Print and shaded views of the part. All mm, measured from the part's lowest x, y and z. A direction names the side the tool comes from. Round coordinates to 2 decimals unless told otherwise and drop trailing zeros. Order: outer loops, then holes, each group sorted by start corner. A loop starts at its lowest first (then second) coordinate and runs counter-clockwise, first axis right, second up. Notation, with made-up numbers: (77, 32) -> (123, 32) arc R26 cw to (123, 69) -> close; hole circle Ø1 at (10.5, 68.25). An arc over 180 degrees is marked (long way). Answer as CSV lines item,"result".
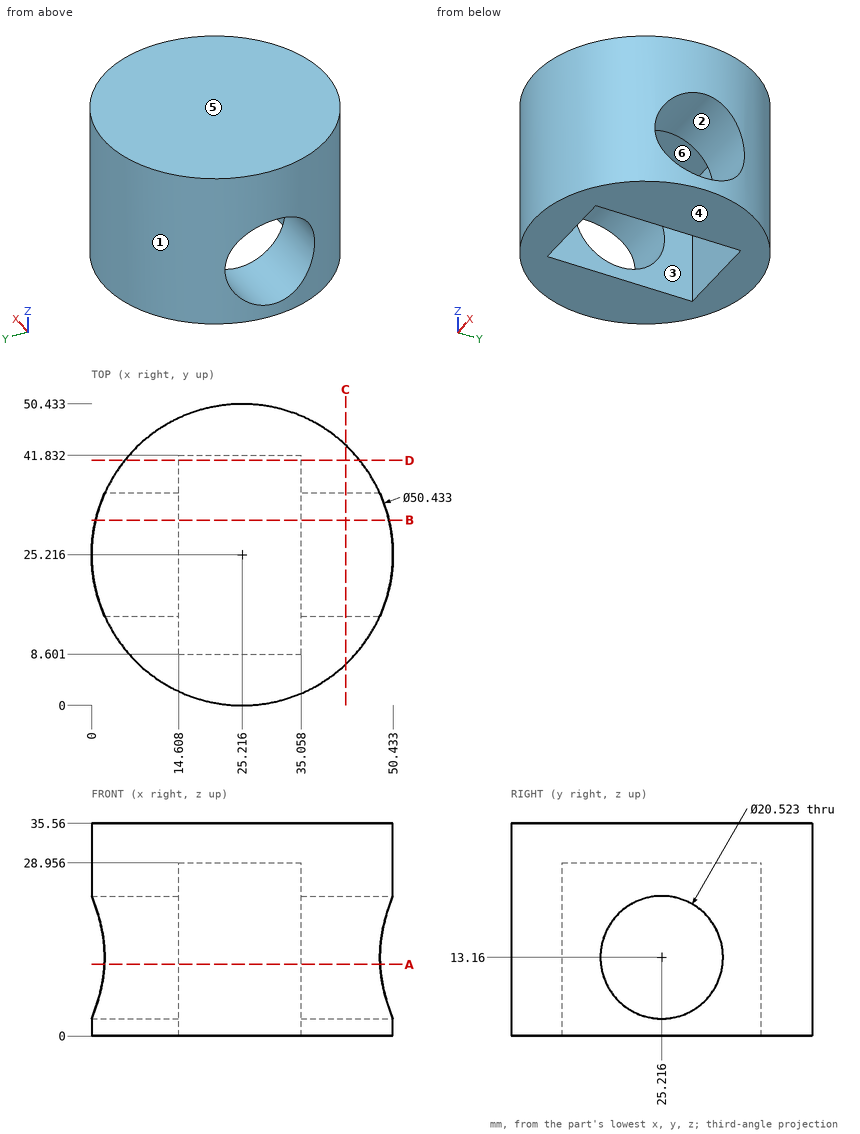
Q1. Mould opens along Y. For the marked faces 1, 2, 3 and 4 say: +Y half, -Y half, draft (parallel to the pull), parting line (faces both ways), or undercut.
Checks:
face 1,"parting line"
face 2,"undercut"
face 3,"undercut"
face 4,"draft"
Q2. Saw through at B-B (y = 31). Write the cut outline in (x, z).
Checks:
outline,"(0.67, 0) -> (14.61, 0) -> (14.61, 4.68) -> (0.67, 4.68) -> close; (0.67, 21.64) -> (14.61, 21.64) -> (14.61, 28.96) -> (35.06, 28.96) -> (35.06, 21.64) -> (49.76, 21.64) -> (49.76, 35.56) -> (0.67, 35.56) -> close; (35.06, 0) -> (49.76, 0) -> (49.76, 4.68) -> (35.06, 4.68) -> close"
Q3. Saw through at D-D (y = 41). Write the cut outline in (x, z).
Checks:
outline,"(5.55, 0) -> (14.61, 0) -> (14.61, 28.96) -> (35.06, 28.96) -> (35.06, 0) -> (44.88, 0) -> (44.88, 35.56) -> (5.55, 35.56) -> close"
Q4. Wall check: L1, parallel to Z at x = 25.5, y = 20.5; L2, parallel to Y at x = 16, z = 25 (1 decimal); L3, parallel to X at y = 23, z = 25.5 (1 decimal). Give the ranges that are in metal, low to high. Write a range as [from, to].
Checks:
L1,"[28.96, 35.56]"
L2,"[1.7, 8.6], [41.8, 48.7]"
L3,"[0.1, 14.6], [35.1, 50.3]"
Q5. Saw through at C-C (x = 42.5). Write the cut outline in (y, z) (1 decimal), plus the area to 3 significant figures.
Checks:
outline,"(6.9, 0) -> (43.6, 0) -> (43.6, 35.6) -> (6.9, 35.6) -> close; hole circle Ø20.5 at (25.2, 13.2)"
area,"975 mm²"
Q6. Tool access for the marked faces 5 and 6: list every direction of +Z, -Z, +X, -X, +Y, -Y with a clear straight run to the whole face (end or side of a thin tool).
Checks:
face 5,"+Z, +X, -X, +Y, -Y"
face 6,"-Z"
Q7. Flat gauge pins, fed straight in: pin 1 (4 mm diameter, centred on y = 35.5, z = 30.5, fed in from +X); pin 2 (12 mm diameter, centred on x = 23, z = 16.5, fed in from +Y); pin 3 (1 mm diameter, centred on y = 39, z = 18, fed in from +X). Where does each tip first touch, or does it go through?
Checks:
pin 1,"x = 49.03"
pin 2,"y = 50.43"
pin 3,"x = 46.65"
Q8. Saw through at A-A (z = 12). Write the cut outline in (x, y).
Checks:
outline,"(2.15, 15.02) arc R25.22 ccw to (48.28, 15.02) -> (35.06, 15.02) -> (35.06, 8.6) -> (14.61, 8.6) -> (14.61, 15.02) -> close; (2.15, 35.41) -> (14.61, 35.41) -> (14.61, 41.83) -> (35.06, 41.83) -> (35.06, 35.41) -> (48.28, 35.41) arc R25.22 ccw to start"
